Read the model definition and answer for the solid it produces. Units are mm, in the model's axes. Face numbers are marked on the shaded views. Coordinates: 2 decimals unless noted, no trailing zeros. Write each loop counter-clockwise with the first axis right and the second up, starting at its lowest first coordinate (ties: lowest second). Pieces come first, ordered by that corner, then holes. Notation, with made-up numbers: (-11.75, 1) -> (22.25, 1) arc R14 cw to (22.25, 20) -> close; hole circle Ø11 at (18.25, 76.25). An arc over 180 degrees is marked (long way). Answer in a Markdown table with one row per item. Add a question column.
Item 1: Section C-C on x = 178 is taken. Write down the section's boundary in (y, z).
Item 2: Straight lines are drawn through the part: line 1 (X direction, y = 0, z = 125); line 2 (Y direction, x = 178, z = 136); line 3 (Y direction, x = 234.5, z = -7). For each, find the intervals that lie inside material, in ascending order. Write a range as from..to.
Item 3: Section B-B on y = 0 is taken. Write down the section's boundary in (x, z).
Item 4: Section A-A on z = 0 is taken. Write down the section's boundary in (x, y), then the cut area to 3 significant figures.
Item 5: For a pull along Z with two mould halves and no side action, classify the marked faces 1 and 2 as +Z half, -Z half, draft (parallel to the pull), parting line (faces both ways), or undercut.
Item 6: Section D-D on x = 55 is taken. Write down the section's boundary in (y, z), then the cut area to 3 significant figures.
Item 7: Given pin 1 Ø1.5 at (x, z) = (179, -79) entering from -Y; pin 2 Ø4 at (x, z) = (306.5, -61.5) entering from +Y; pin 3 Ø1 at (x, z) = (134.5, -57) entering from -Y, each flat-ended and moving along its own axis, determine where each tip first touches the part or whether it passes through.
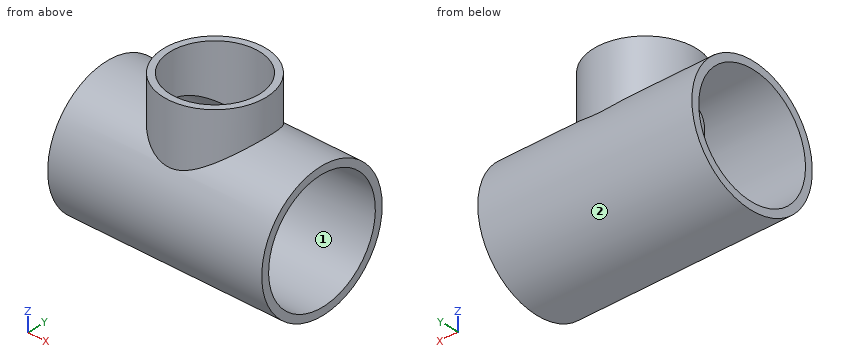
Autodesk Inventor part; units mm, degrees
ref_plane "YZ Plane" through (0, 0, 0) normal (1, 0, 0) x (0, 1, 0)
ref_plane "XZ Plane" through (0, 0, 0) normal (0, 1, 0) x (-1, 0, 0)
ref_plane "XY Plane" through (0, 0, 0) normal (0, 0, 1) x (1, 0, 0)
sketch "Sketch1" plane through (0, 0, 0) normal (1, 0, 0) x (0, 1, 0)
  circle A0 centre (0, 0) radius 109.55
  dimension "d0" = 219.1
extrude "Extrude1" add sketch "Sketch1" along normal blind 356
sketch "Sketch2" plane through (0, 0, 0) normal (0, 0, 1) x (1, 0, 0)
  line L0 (0, 109.55) -> (0, -109.55)
  line L1 (356, 109.55) -> (356, -109.55)
  line L2 (0, 0) -> (356, 0) construction
  circle A0 centre (178, 0) radius 84.15
  dimension "d3" = 168.3
extrude "Extrude2" add sketch "Sketch2" along normal blind 168
sketch "Sketch3" plane through (0, 0, 0) normal (-1, 0, 0) x (0, 0, 1)
  circle A0 centre (0, 0) radius 109.55
  circle A1 centre (0, 0) radius 97.05
  dimension "a" = 178
  dimension "d6" = 194.1
extrude "Extrude3" cut sketch "Sketch3" against normal through all contours A1
sketch "Sketch4" plane through (178, 0, 168) normal (0, 0, 1) x (1, 0, 0)
  circle A0 centre (0, 0) radius 84.15
  circle A1 centre (0, 0) radius 73.15
  dimension "d9" = 146.3
extrude "Extrude4" cut sketch "Sketch4" against normal up to next contours A1
equation "\"d0\" = D1"
equation "\"d1\" = 2 * a"
equation "\"d3\" = D2"
equation "\"d4\" = b"
equation "\"a\" = 178"
equation "\"d6\" = D1 - 2 * s1"
equation "\"d7\" = a"
equation "\"d9\" = D2 - 2 * s2"
equation "\"d10\" = a"
equation "\"D1\" = 219.1"
equation "\"s1\" = 12.5"
equation "\"D2\" = 168.3"
equation "\"s2\" = 11"
equation "\"b\" = 168"
equation "\"Size_Designation\" = 1.2345"
properties part number "DIN 2615-1 Reducing Tee 219.1 x 12.5 - 168.3 x 11 S" material "Steel"
Results below:
| question | item | result |
|---|---|---|
| 1 | outline | (-84.15, 70.14) arc R109.55 ccw (long way) to (84.15, 70.14) -> (84.15, 168) -> (73.15, 168) -> (73.15, 63.78) arc R97.05 cw (long way) to (-73.15, 63.78) -> (-73.15, 168) -> (-84.15, 168) -> close |
| 2 | line 1 | x = 93.85..104.85, 251.15..262.15 |
| 2 | line 2 | y = -84.15..-73.15, 73.15..84.15 |
| 2 | line 3 | y = -109.33..-96.8, 96.8..109.33 |
| 3 | outline | (0, -109.55) -> (356, -109.55) -> (356, -97.05) -> (0, -97.05) -> close; (0, 97.05) -> (104.85, 97.05) -> (104.85, 168) -> (93.85, 168) -> (93.85, 109.55) -> (0, 109.55) -> close; (251.15, 97.05) -> (356, 97.05) -> (356, 109.55) -> (262.15, 109.55) -> (262.15, 168) -> (251.15, 168) -> close |
| 4 | outline | (0, -109.55) -> (356, -109.55) -> (356, -97.05) -> (0, -97.05) -> close; (0, 97.05) -> (356, 97.05) -> (356, 109.55) -> (0, 109.55) -> close |
| 4 | area | 8,900 mm2 |
| 5 | face 1 | undercut |
| 5 | face 2 | parting line |
| 6 | outline | circle Ø219.1 at (0, 0); hole circle Ø194.1 at (0, 0) |
| 6 | area | 8,110 mm2 |
| 7 | pin 1 | stops at y = -76.67 |
| 7 | pin 2 | stops at y = 91.98 |
| 7 | pin 3 | stops at y = -93.86 |
